```python
from build123d import *

# Parameters (mm, degrees)
SKETCH_1_W          = 49.3
SKETCH_1_H          = 15
EXTRUDE_1_DEPTH     = 3
SKETCH_2_W          = 5
SKETCH_2_H          = 4.567504656
SKETCH_2_H_2        = 2.332495344
EXTRUDE_2_DEPTH     = 5.5
SKETCH_3_R          = 0.75
EXTRUDE_3_DEPTH     = 1.5
SKETCH_4_R          = 1
CUT_EXTRUDE_1_DEPTH = 10
CUT_EXTRUDE_2_DEPTH = 4
EXTRUDE_4_DEPTH     = 3
SKETCH_9_R          = 1
EXTRUDE_5_DEPTH     = 4.5
EXTRUDE_9_DEPTH     = 4
SKETCH_8_R          = 1.6
CUT_EXTRUDE_3_DEPTH = 56.068502794
CUT_EXTRUDE_4_DEPTH = 2.3
SKETCH_13_W         = 3.2
SKETCH_13_H         = 6.4
CUT_EXTRUDE_5_DEPTH = 1.2


with BuildPart() as part:
    # 草图1 → 凸台-拉伸1 (new body)
    with BuildSketch(Plane.XY):
        with Locations((24.65, 7.5)):
            Rectangle(SKETCH_1_W, SKETCH_1_H)
    extrude(amount=EXTRUDE_1_DEPTH)

    # 草图2 → 凸台-拉伸2 (add)
    with BuildSketch(Plane.XY.offset(3)):
        Polygon((7.75, 6.9), (7.75, 15), (0, 15), (0, 0), (11.25, 0), (11.25, 6.9), align=None)
        with Locations((20.4, 2.283752328)):
            Rectangle(SKETCH_2_W, SKETCH_2_H)
        with Locations((20.4, 5.733752328)):
            Rectangle(SKETCH_2_W, SKETCH_2_H_2)
        Polygon((49.3, 15), (33.05, 15), (33.05, 6.9), (29.55, 6.9), (29.55, 0), (49.3, 0), align=None)
    extrude(amount=EXTRUDE_2_DEPTH)

    # 草图3 → 凸台-拉伸3 (add)
    with BuildSketch(Plane.XY.offset(3)):
        with Locations((10.15, 11)):
            Circle(SKETCH_3_R)
        with Locations((30.65, 11)):
            Circle(SKETCH_3_R)
    extrude(amount=EXTRUDE_3_DEPTH)

    # 草图4 → 切除-拉伸1 (cut)
    with BuildSketch(Plane.XY.offset(8.5)):
        with Locations((3.875, 7.5)):
            Circle(SKETCH_4_R)
        with Locations((41.175, 7.5)):
            Circle(SKETCH_4_R)
    extrude(amount=-CUT_EXTRUDE_1_DEPTH, mode=Mode.SUBTRACT)

    # 草图5 → 切除-拉伸2 (cut)
    with BuildSketch(Plane(origin=(0, 0, 0), x_dir=(-1, 0, 0), z_dir=(0, 0, -1))):
        Polygon((-5.000833025, 9.45), (-6.12666605, 7.5), (-5.000833025, 5.55), (-2.749166975, 5.55), (-1.62333395, 7.5), (-2.749166975, 9.45), align=None)
        Polygon((-42.300833025, 9.45), (-43.42666605, 7.5), (-42.300833025, 5.55), (-40.049166975, 5.55), (-38.92333395, 7.5), (-40.049166975, 9.45), align=None)
    extrude(amount=-CUT_EXTRUDE_2_DEPTH, mode=Mode.SUBTRACT)

    # 草图6 → 凸台-拉伸4 (add)
    with BuildSketch(Plane.ZY):
        with BuildLine():
            Line((2.6, 6), (2.6, 12))
            ThreePointArc((2.6, 12), (4, 13.4), (5.4, 12))
            Line((5.4, 12), (5.4, 6))
            ThreePointArc((5.4, 6), (4, 4.6), (2.6, 6))
        make_face()
    extrude_4 = extrude(amount=EXTRUDE_4_DEPTH)

    # 镜向1: 凸台-拉伸4 across plane
    add(extrude_4.mirror(Plane.ZY.offset(-24.65)))

    # 草图9 → 凸台-拉伸5 (add)
    with BuildSketch(Plane.XY.offset(8.5)):
        with Locations((41.175, 7.5)):
            Circle(SKETCH_9_R)
        with Locations((3.875, 7.5)):
            Circle(SKETCH_9_R)
    extrude(amount=-EXTRUDE_5_DEPTH)

    # 草图10 → 凸台-拉伸9 (add)
    with BuildSketch(Plane(origin=(0, 0, 0), x_dir=(-1, 0, 0), z_dir=(0, 0, -1))):
        Polygon((-2.749166975, 9.45), (-5.000833025, 9.45), (-6.12666605, 7.5), (-5.000833025, 5.55), (-2.749166975, 5.55), (-1.62333395, 7.5), align=None)
        Polygon((-40.049166975, 9.45), (-42.300833025, 9.45), (-43.42666605, 7.5), (-42.300833025, 5.55), (-40.049166975, 5.55), (-38.92333395, 7.5), align=None)
    extrude(amount=-EXTRUDE_9_DEPTH)

    # 草图8 → 切除-拉伸3 (cut, through all)
    with BuildSketch(Plane.XY.offset(8.5)):
        with Locations((5.75, 7.5)):
            Circle(SKETCH_8_R)
        with Locations((37.3, 7.5)):
            Circle(SKETCH_8_R)
    extrude(amount=-CUT_EXTRUDE_3_DEPTH, mode=Mode.SUBTRACT)

    # 草图11 → 切除-拉伸4 (cut)
    with BuildSketch(Plane(origin=(0, 0, 0), x_dir=(-1, 0, 0), z_dir=(0, 0, -1))):
        Polygon((-37.3, 10.617691454), (-40, 9.058845727), (-40, 5.941154273), (-37.3, 4.382308546), (-34.6, 5.941154273), (-34.6, 9.058845727), align=None)
        Polygon((-5.75, 10.617691454), (-8.45, 9.058845727), (-8.45, 5.941154273), (-5.75, 4.382308546), (-3.05, 5.941154273), (-3.05, 9.058845727), align=None)
    extrude(amount=-CUT_EXTRUDE_4_DEPTH, mode=Mode.SUBTRACT)

    # 草图13 → 切除-拉伸5 (cut)
    with BuildSketch(Plane.XY.offset(8.5)):
        with Locations((1.6, 8.65)):
            Rectangle(SKETCH_13_W, SKETCH_13_H)
    cut_extrude_5 = extrude(amount=-CUT_EXTRUDE_5_DEPTH, mode=Mode.SUBTRACT)

    # 镜向2: 切除-拉伸5 across plane
    add(cut_extrude_5.mirror(Plane.ZY.offset(-24.65)), mode=Mode.SUBTRACT)


solid = part.part
```
Verification items for the finished model (mm, model axes). A direction names the side the tool comes from. Give positions to 0.01 mm unless a question says otherwise; leave off trailing zeros. Order: outer loops, then holes, each group sorted by start corner. A loop starts at its lowest first (then second) coordinate and runs counter-clockwise, first axis right, second up. Notation, with made-up numbers: (-29, 16.5) - (-21, 16.5) arc R20 ccw to (-21, 47.5) - close; hole circle Ø4 at (10.5, 26). An arc over 180 degrees is marked (long way). Answer as CSV lines item,"result". Start each with the question number.
Item 1: Section check C-C, the plane y = 1.5. Record the boundary of the cut face in (x, z).
Item 2: Material ranges on L1, parallel to X at y = 2, z = 3.5; L2, parallel to X at y = 6.5, z = 0.5; L3, parallel to Y at x = 37.3, z = 4.75, recorded low to high.
Item 3: Access from +Z, -Z, +X, -X, +Y, -Y to the whole of each face (thin tool, end or side, straight path). Record for faces 4 (the face through (33.05, 11, 6)), 5 (the face through (-1.5, 13.4, 4)), 6 (the face through (-1, 9, 5.4)), 7 (the face through (4.42, 5.15, 1.13)).
Item 4: Mould release check, pull along X, two halves, no side actions. Record for faces 1 (the face through (-1, 9, 2.6)), 2 (the face through (30.1, 11.51, 3.74)), 3 (the face through (46.1, 9, 8)): released by +X, released by -X, zero draft, split by the parting line, or undercut.
Item 5: Section check B-B, the plane z = 4. Record the boundary of the cut face in (x, y), plus the area to 3 significant figures.
Item 6: Gauge pin test, flat ends, axial feed: pin 1 (4.5 mm diameter, centred on y = 2, z = 4.5, fed in from +X); pin 2 (1.6 mm diameter, centred on x = 7, y = 6.5, fed in from -Z); pin 3 (0.6 mm diameter, centred on y = 8.5, z = 7.5, fed in from -X). Record the tip position at first contact, or that the pin passes through.
Item 7: Section check D-D, the plane y = 7.5. State how many separate pieces and enclosed holes the cut face has, plus the area to 4 significant figures.
Item 8: Section check A-A, the plane z = 6.75. Record the boundary of the cut face in (x, y), plus the area to 3 significant figures.
Filled in:
1,outline,"(0, 0) - (49.3, 0) - (49.3, 8.5) - (29.55, 8.5) - (29.55, 3) - (22.9, 3) - (22.9, 8.5) - (17.9, 8.5) - (17.9, 3) - (11.25, 3) - (11.25, 8.5) - (0, 8.5) - close"
2,L1,"0 to 11.25, 17.9 to 22.9, 29.55 to 49.3"
2,L2,"0 to 3.05, 8.45 to 34.6, 40 to 49.3"
2,L3,"0 to 5.9, 9.1 to 15"
3,face 4,"+Z, +Y"
3,face 5,"-X, +Y"
3,face 6,"+Z, -X, +Y, -Y"
3,face 7,"-Z"
4,face 1,"zero draft"
4,face 2,"undercut"
4,face 3,"released by +X"
5,outline,"(-3, 4.6) - (0, 4.6) - (0, 0) - (11.25, 0) - (11.25, 6.9) - (7.75, 6.9) - (7.75, 15) - (0, 15) - (0, 13.4) - (-3, 13.4) - close; circle Ø1.5 at (10.15, 11); (17.9, 0) - (22.9, 0) - (22.9, 6.9) - (17.9, 6.9) - close; (29.55, 0) - (49.3, 0) - (49.3, 4.6) - (52.3, 4.6) - (52.3, 13.4) - (49.3, 13.4) - (49.3, 15) - (33.05, 15) - (33.05, 6.9) - (29.55, 6.9) - close; circle Ø1.5 at (30.65, 11); hole circle Ø3.2 at (5.75, 7.5); hole circle Ø3.2 at (37.3, 7.5)"
5,area,"483 mm^2"
6,pin 1,"x = 49.3"
6,pin 2,"z = 2.3"
6,pin 3,"x = 0"
7,separate pieces,"3"
7,enclosed holes,"0"
7,area,"224.5 mm^2"
8,outline,"(0, 0) - (11.25, 0) - (11.25, 6.9) - (7.75, 6.9) - (7.75, 15) - (0, 15) - close; (17.9, 0) - (22.9, 0) - (22.9, 6.9) - (17.9, 6.9) - close; (29.55, 0) - (49.3, 0) - (49.3, 15) - (33.05, 15) - (33.05, 6.9) - (29.55, 6.9) - close; hole circle Ø3.2 at (5.75, 7.5); hole circle Ø3.2 at (37.3, 7.5)"
8,area,"427 mm^2"
